Source: CAD feature listing. Evaluate the final solid. Frame: model axes, mm. A direction names the side the tool comes from. Give positions to 0.01 mm unless a question says otherwise; leave off trailing zeros. Loops run counter-clockwise (first coordinate to the right, second up) from the corner with the lowest first, then second, coordinate; pieces in that order, holes last. Notation, with made-up numbers: (44, -14) - (69, -14) arc R11 ccw to (69, -9) - close; hole circle Ø3 at (8, -12). An arc over 180 degrees is marked (long way). Put each result on its own line as item: value.
Autodesk Inventor part; units mm, degrees
ref_plane "YZ Plane" through (0, 0, 0) normal (1, 0, 0) x (0, 1, 0)
ref_plane "XZ Plane" through (0, 0, 0) normal (0, 1, 0) x (-1, 0, 0)
ref_plane "XY Plane" through (0, 0, 0) normal (0, 0, 1) x (1, 0, 0)
sketch "Boceto1" plane through (0, 0, 0) normal (0, 1, 0) x (-1, 0, 0)
  line L0 (-19.9533, 14.4643) -> (7.0467, 14.4643)
  line L1 (7.0467, 14.4643) -> (7.0467, -12.5357)
  line L2 (7.0467, -12.5357) -> (-19.9533, -12.5357)
  line L3 (-19.9533, -12.5357) -> (-19.9533, 14.4643)
  point P0 (0, 0)
  dimension "d0" = 27
  dimension "d1" = 27
extrude "Extrusión1" add sketch "Boceto1" along normal blind 62
sketch "Boceto2" plane through (0, 62, 0) normal (0, 1, 0) x (1, 0, 0)
  line L0 (-7.0467, -14.4643) -> (19.9533, -14.4643)
  line L1 (19.9533, -14.4643) -> (19.9533, 12.5357)
  line L2 (19.9533, 12.5357) -> (-7.0467, 12.5357)
  line L3 (-7.0467, 12.5357) -> (-7.0467, -14.4643)
  line L4 (-1.0467, 6.5357) -> (13.9533, 6.5357)
  line L5 (13.9533, 6.5357) -> (13.9533, -8.4643)
  line L6 (13.9533, -8.4643) -> (-1.0467, -8.4643)
  line L7 (-1.0467, -8.4643) -> (-1.0467, 6.5357)
  point P0 (0, 0)
  dimension "d4" = 6
  dimension "d5" = 6
  dimension "d6" = 6
  dimension "d7" = 6
extrude "Extrusión2" cut sketch "Boceto2" against normal blind 31 contours L4 L5 L6 L7
sketch "Boceto3" plane through (19.9533, 0, -12.5357) normal (0, 0, -1) x (-1, 0, 0)
  line L0 (27, 0) -> (0, 0)
  line L1 (27, 0) -> (27, 62)
  line L2 (0, 0) -> (0, 62)
  line L3 (20, 25) -> (7, 25)
  line L4 (7, 25) -> (7, 0)
  line L5 (7, 0) -> (20, 0)
  line L6 (20, 0) -> (20, 25)
  line L7 (0, 62) -> (27, 62)
  circle A0 centre (13.5, 39) radius 2.55
  point P0 (19.9533, 0)
  dimension "d10" = 7
  dimension "d11" = 7
  dimension "d12" = 25
  dimension "d16" = 5.1
  dimension "d17" = 13.5
  dimension "d18" = 23
extrude "Extrusión3" cut sketch "Boceto3" against normal blind 30 contours L0 L4 L3 L6
sketch "Boceto4" plane through (19.9533, 62, -12.5357) normal (0, 0, -1) x (-1, 0, 0)
  line L0 (0, -62) -> (0, 0)
  circle A0 centre (13.5, -25) radius 1.55
  line L1 (21, -31) -> (6, -31)
  point P0 (19.9533, -62)
  dimension "d19" = 3.1
  dimension "d20" = 13.5
  dimension "d34" = 6
extrude "Extrusión4" cut sketch "Boceto4" against normal blind 7
sketch "Boceto5" plane through (-7.0467, 62, 14.4643) normal (0, 0, 1) x (1, 0, 0)
  line L0 (27, -62) -> (27, 0)
  circle A0 centre (13.5, -25) radius 7.75
  line L1 (21, -31) -> (6, -31)
  point P0 (7.0467, -62)
  dimension "d24" = 15.5
  dimension "d25" = 13.5
  dimension "d33" = 6
extrude "Extrusión5" cut sketch "Boceto5" against normal blind 3
sketch "Boceto6" plane through (6.4533, 37, 11.4643) normal (0, 0, 1) x (1, 0, 0)
  circle A0 centre (0, 0) radius 7.75
  circle A1 centre (0, 0) radius 5.65
  point P0 (-6.4533, -37)
  dimension "d29" = 11.3
extrude "Extrusión6" cut sketch "Boceto6" against normal blind 3 contours A1
sketch "Boceto8" plane through (-7.0467, 0, -12.5357) normal (-1, 0, 0) x (0, 0, 1)
  line L0 (27, 0) -> (27, 62)
  circle A0 centre (13.5, 37) radius 1.5
  line L1 (0, 25) -> (27, 25)
  line L2 (0, 25) -> (27, 25)
  point P0 (12.5357, 0)
  dimension "d42" = 13.5
  dimension "d43" = 3
  dimension "d47" = 12
extrude "Extrusión8" cut sketch "Boceto8" against normal through all
sketch "Boceto9" plane through (0, 62, 0) normal (0, 1, 0) x (1, 0, 0)
  line L0 (-7.0467, -14.4643) -> (19.9533, -14.4643)
  line L1 (19.9533, -14.4643) -> (19.9533, 12.5357)
  line L2 (19.9533, 12.5357) -> (-7.0467, 12.5357)
  line L3 (-7.0467, 12.5357) -> (-7.0467, -14.4643)
  circle A0 centre (-3.5467, 9.0357) radius 1.5
  circle A1 centre (16.4533, 9.0357) radius 1.5
  circle A2 centre (-3.5467, -10.9643) radius 1.5
  circle A3 centre (16.4533, -10.9643) radius 1.5
  point P0 (0, 0)
  dimension "d48" = 3
  dimension "d49" = 3.5
  dimension "d50" = 3.5
  dimension "d51" = 3.5
  dimension "d52" = 3.5
  dimension "d53" = 3
  dimension "d54" = 3
  dimension "d55" = 3.5
  dimension "d56" = 3.5
  dimension "d57" = 3.5
  dimension "d58" = 3.5
  dimension "d59" = 3
extrude "Extrusión9" cut sketch "Boceto9" against normal blind 6 contours A0 | A1 | A2 | A3
sketch "Boceto10" plane through (0, 31, 0) normal (0, 1, 0) x (1, 0, 0)
  line L0 (-1.0467, 6.5357) -> (13.9533, 6.5357)
  line L1 (13.9533, 6.5357) -> (13.9533, -8.4643)
  circle A0 centre (6.4533, -0.9643) radius 1.5
  point P0 (0, 0)
  dimension "d62" = 3
  dimension "d63" = 7.5
  dimension "d64" = 7.5
extrude "Extrusión10" cut sketch "Boceto10" against normal through all
properties part number "Cubeta Final"
1) Material intervals for line 1 along X through (y, z) = (18.5, 12); line 2 along X through (y, z) = (52.5, 5); line 3 along Y through (x, z) = (12.75, -4.75), sorted ascending. Write a range as [from, to].
Check result:
line 1: [-7.05, -0.05], [12.95, 19.95]
line 2: [-7.05, -1.05], [13.95, 19.95]
line 3: [25, 31]
2) Section query C-C, the plane y = 24. Output: boundary loops of the cut face in (x, z), plus the area to 3 significant figures.
Check result:
outline: (-7.05, -12.54) - (-0.05, -12.54) - (-0.05, 14.46) - (-7.05, 14.46) - close; (12.95, -12.54) - (19.95, -12.54) - (19.95, 14.46) - (12.95, 14.46) - close
area: 378 mm²
3) Mould query, pull axis X, two halves, no side actions, for faces 4 (the cylindrical face through (6.789, 35.487, -9.578)), 5 (the flat face through (-7.047, 31, 1)), 6 (the flat face through (-2, 62, 1)), 7 (the flat face through (12.953, 13, 1)). Classes: pulls with the +X half, pulls with the -X half, needs draft (parallel to the pull), parting line crosses it, or undercut.
Check result:
face 4: undercut
face 5: pulls with the -X half
face 6: needs draft
face 7: undercut
4) Section query A-A, the plane y = 37. Output: boundary loops of the cut face in (x, z), plus the area to 3 significant figures.
Check result:
outline: (-7.05, -12.54) - (4.9, -12.54) - (4.9, -6.54) - (-1.05, -6.54) - (-1.05, -0.54) - (-7.05, -0.54) - close; (-7.05, 2.46) - (-1.05, 2.46) - (-1.05, 8.46) - (0.8, 8.46) - (0.8, 11.46) - (-1.3, 11.46) - (-1.3, 14.46) - (-7.05, 14.46) - close; (8, -12.54) - (19.95, -12.54) - (19.95, -0.54) - (13.95, -0.54) - (13.95, -6.54) - (8, -6.54) - close; (12.1, 8.46) - (13.95, 8.46) - (13.95, 2.46) - (19.95, 2.46) - (19.95, 14.46) - (14.2, 14.46) - (14.2, 11.46) - (12.1, 11.46) - close
area: 369 mm²
5) Pin query (flat end, axial travel): P1, Ø12, axis at x = 7, z = -0.5, coming from the +Y side; P2, Ø1.5, axis at x = 9.5, z = -7, coming from the -Y side; P3, Ø2.5, axis at x = -3.55, z = -9.04, coming from the +Y side; P4, Ø2.5, axis at y = 37, z = 0.96, coming from the +X side. Return the tip coordinate at first contact, or that it passes through.
Check result:
P1: y = 31
P2: y = 25
P3: y = 56
P4: through
6) Section query D-D, the plane y = 46.5. Output: boundary loops of the cut face in (x, z).
Check result:
outline: (-7.05, -12.54) - (19.95, -12.54) - (19.95, 14.46) - (-7.05, 14.46) - close; hole (-1.05, -6.54) - (13.95, -6.54) - (13.95, 8.46) - (-1.05, 8.46) - close
7) Access query for faces 1 (the flat face through (7, 50, 8.464)), 2 (the flat face through (3, 25, 1)), 3 (the cylindrical face through (16.911, 35.536, 0.639)). Directions: +Z, -Z, +X, -X, +Y, -Y. A direction counts if a zero-diameter tool reaches every point of the face in a straight line with its end or side. Return the directions, or none.
Check result:
face 1: +Y
face 2: +Z, -Z, -Y
face 3: +X, -X
8) Section query B-B, the plane x = 7. Output: boundary loops of the cut face in (y, z), plus the area to 3 significant figures.
Check result:
outline: (25, -12.54) - (35.55, -12.54) - (35.55, -6.54) - (31, -6.54) - (31, -0.43) - (25, -0.43) - close; (25, 2.36) - (31, 2.36) - (31, 8.46) - (31.38, 8.46) - (31.38, 11.46) - (29.27, 11.46) - (29.27, 14.46) - (25, 14.46) - close; (38.45, -12.54) - (62, -12.54) - (62, -6.54) - (38.45, -6.54) - close; (42.62, 8.46) - (62, 8.46) - (62, 14.46) - (44.73, 14.46) - (44.73, 11.46) - (42.62, 11.46) - close
area: 420 mm²
